Geometry: final body of the model. Coordinates: model frame, mm. Face numbers are marked on the shaded views. A direction names the side the tool comes from. Give positions to 0.01 mm unless a question says otherwise; leave off trailing zeros. Loops run counter-clockwise (first coordinate to the right, second up) from the corner with the lowest first, then second, coordinate; pieces in that order, holes last. Notation, with made-up numbers: (3, 16.25) - (19, 16.25) arc R25 ccw to (19, 31.25) - close; hole circle Ø3 at (72, 79). An arc over 180 degrees is marked (long way). Answer in a Markdown table with one row per item.
from build123d import *

# Parameters (mm, degrees)
SKETCH_R        = 24.499989
PAD_DEPTH       = 6.5
SKETCH001_R     = 12
PAD001_DEPTH    = 22.4
SKETCH002_R     = 10
POCKET_DEPTH    = 30
SKETCH003_R     = 21.680004
POCKET001_DEPTH = 4.5
FILLET_R        = 2
FILLET001_R     = 1
FILLET002_R     = 1


with BuildPart() as part:
    # Sketch → Pad (new body)
    with BuildSketch(Plane.XY):
        Circle(SKETCH_R)
    extrude(amount=PAD_DEPTH)

    # Sketch001 (on Face3 of Pad) → Pad001 (join)
    with BuildSketch(Plane.XY.offset(6.5)):
        Circle(SKETCH001_R)
    extrude(amount=PAD001_DEPTH)

    # Sketch002 (on Face5 of Pad001) → Pocket (cut)
    with BuildSketch(Plane.XY.offset(28.9)):
        Circle(SKETCH002_R)
    extrude(amount=-POCKET_DEPTH, mode=Mode.SUBTRACT)

    # Sketch003 (on Face2 of Pocket) → Pocket001 (cut)
    with BuildSketch(Plane(origin=(0, 0, 0), x_dir=(1, 0, 0), z_dir=(0, 0, -1))):
        Circle(SKETCH003_R)
    extrude(amount=-POCKET001_DEPTH, mode=Mode.SUBTRACT)

    # Fillet
    fillet_edges = [part.edges().sort_by_distance(p)[0] for p in [
        (-10, 0, 4.5),
    ]]
    fillet(fillet_edges, radius=FILLET_R)

    # Fillet001
    fillet001_edges = [part.edges().sort_by_distance(p)[0] for p in [
        (-24.499989, 0, 6.5),
    ]]
    fillet(fillet001_edges, radius=FILLET001_R)

    # Fillet002
    fillet002_edges = [part.edges().sort_by_distance(p)[0] for p in [
        (-12, 0, 6.5),
    ]]
    fillet(fillet002_edges, radius=FILLET002_R)


solid = part.part
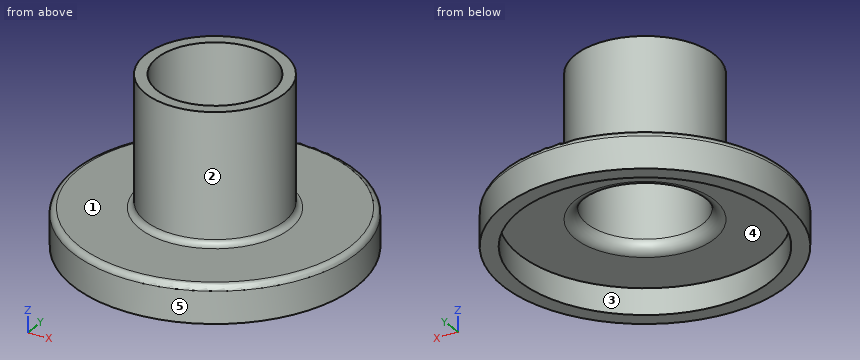
Q1. Material intervals for line 1 along Z through (x, y) = (-20, 8.5); line 2 along Y through (x, z) = (1, 2.75); line 3 along Z through (x, y) = (-17, -3), sorted ascending.
Check values:
| item | result |
|---|---|
| line 1 | 0 to 6.5 |
| line 2 | -24.48 to -21.66, 21.66 to 24.48 |
| line 3 | 4.5 to 6.5 |
Q2. Cut plane A-A (y = 0). Output: boundary loops of the cut face in (x, z), and give its area (3 significant figures).
Check values:
| item | result |
|---|---|
| outline | (-24.5, 0) - (-21.68, 0) - (-21.68, 4.5) - (-12, 4.5) arc R2 ccw to (-10, 6.5) - (-10, 28.9) - (-12, 28.9) - (-12, 7.5) arc R1 cw to (-13, 6.5) - (-23.5, 6.5) arc R1 ccw to (-24.5, 5.5) - close; (10, 6.5) arc R2 ccw to (12, 4.5) - (21.68, 4.5) - (21.68, 0) - (24.5, 0) - (24.5, 5.5) arc R1 ccw to (23.5, 6.5) - (13, 6.5) arc R1 cw to (12, 7.5) - (12, 28.9) - (10, 28.9) - close |
| area | 171 mm² |
Q3. Reachability of the marked faces 4 and 5 from +Z, -Z, +X, -X, +Y, -Y: full face, straight path, thin tool, end or side. Return the list, or none.
Check values:
| item | result |
|---|---|
| face 4 | -Z |
| face 5 | +Z, -Z |
Q4. Cut plane C-C (z = 13). Output: boundary loops of the cut face in (x, y).
Check values:
| item | result |
|---|---|
| outline | circle Ø24 at (0, 0); hole circle Ø20 at (0, 0) |
Q5. Draft query along X for the marked faces 1, 2 and 3. Return one class per face: pulls with the +X half, pulls with the -X half, needs draft (parallel to the pull), parting line crosses it, or undercut.
Check values:
| item | result |
|---|---|
| face 1 | needs draft |
| face 2 | parting line crosses it |
| face 3 | undercut |
Q6. First-contact query: pin 1 (8 mm diameter, centred on x = -8, y = -18.5, fed in from -Z); pin 2 (12 mm diameter, centred on x = -0.5, z = 24, fed in from -Y); pin 3 (16 mm diameter, centred on x = 0, y = 0, fed in from -Z); pin 4 (21.5 mm diameter, centred on x = 4, y = -6, fed in from -Z). Flat tips, straight axial feed; report the tip coordinate or a pass-through.
Check values:
| item | result |
|---|---|
| pin 1 | z = 0 |
| pin 2 | y = -12 |
| pin 3 | through |
| pin 4 | z = 4.5 |
